```python
from build123d import *

# Parameters (mm, degrees)
F0_W        = 7.62
F0_H        = 17.78
F1_DEPTH    = 12.7
F2_SIZE     = 2.54
F3_R        = 61.3177298103
F4_R        = 76.3155057079
F5_R        = 114.0325409017
F6_T1_DEPTH = 12.7


# Not quite as in the source:
# - a fillet or chamfer that OpenCascade refuses, or shapes differently, is made with other operations: its cross-section is extruded or revolved along the edge and cut away or added


with BuildPart() as f1:
    # F0 (on Front) → F1 (new body)
    with BuildSketch(Plane.XZ):
        with BuildLine():
            Line((-43.3897525072, 184.0122990829), (-43.3897525072, 154.9135648233))
            Line((-43.3897525072, 154.9135648233), (-12.6282460988, 154.9135648233))
            Line((-12.6282460988, 154.9135648233), (-12.6282460988, 184.0122990829))
            Line((-12.6282460988, 184.0122990829), (-23.4354074901, 184.0122990829))
            Line((-23.4354074901, 184.0122990829), (-23.4354074901, 173.8522990829))
            ThreePointArc((-23.4354074901, 173.8522990829), (-24.1793562659, 172.0562478587), (-25.9754074901, 171.3122990829))
            Line((-25.9754074901, 171.3122990829), (-29.7854074901, 171.3122990829))
            ThreePointArc((-29.7854074901, 171.3122990829), (-31.5814587143, 172.0562478587), (-32.3254074901, 173.8522990829))
            Line((-32.3254074901, 173.8522990829), (-32.3254074901, 184.0122990829))
            Line((-32.3254074901, 184.0122990829), (-43.3897525072, 184.0122990829))
        make_face()
        Polygon((-43.3897525072, 154.9135648233), (9.0125808752, 35.5335648233), (34.6665808752, 35.5335648233), (34.6665808752, 53.3135648233), (-12.6282460988, 154.9135648233), align=None)
        with Locations((16.9659831101, 53.1658351564)):
            Rectangle(F0_W, F0_H, mode=Mode.SUBTRACT)
        Polygon((34.6665808752, 35.5335648233), (9.0125808752, 35.5335648233), (9.0125808752, -35.5335648233), (17.9025808752, -35.5335648233), (17.9025808752, 15.2664351767), (25.7765808752, 15.2664351767), (25.7765808752, -35.5335648233), (34.6665808752, -35.5335648233), align=None)
    extrude(amount=F1_DEPTH)

    # F2
    f2_edges = [f1.edges().sort_by_distance(p)[0] for p in [
        (-32.325407, -6.35, 184.012299),
        (-23.435407, -6.35, 184.012299),
        (-12.628246, -6.35, 184.012299),
        (-43.389753, -6.35, 184.012299),
        (17.902581, -6.35, -35.533565),
        (25.776581, -6.35, -35.533565),
        (34.666581, -6.35, -35.533565),
        (9.012581, -6.35, -35.533565),
    ]]
    chamfer(f2_edges, length=F2_SIZE)

    # F3
    f3_edges = [f1.edges().sort_by_distance(p)[0] for p in [
        (34.666581, -6.35, 53.313565),
    ]]
    fillet(f3_edges, radius=F3_R)

    # F4
    f4_edges = [f1.edges().sort_by_distance(p)[0] for p in [
        (-12.628246, -6.35, 154.913565),
    ]]
    fillet(f4_edges, radius=F4_R)

    # F5
    f5_edges = [f1.edges().sort_by_distance(p)[0] for p in [
        (-43.389753, -6.35, 154.913565),
    ]]
    fillet(f5_edges, radius=F5_R)

    # F6: fillet of radius 446.1798259809 on 1 edges, made by hand

    # F6_s2 → F6_t1 (join)
    with BuildSketch(Plane.XZ):
        with BuildLine():
            ThreePointArc((-27.8005344067, 119.3990994032), (-2.6481597508, 44.8323374579), (9.0125808752, -32.9935648233))
            Line((9.0125808752, -32.9935648233), (9.0125808752, 35.5335648233))
            Line((9.0125808752, 35.5335648233), (-27.8005344067, 119.3990994032))
        make_face()
    extrude(amount=F6_T1_DEPTH)


solid = f1.part
```
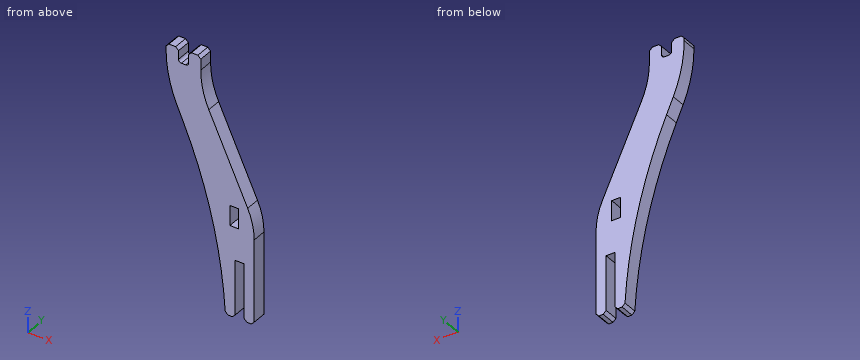
The listing builds one solid part. Answer for the finished solid, in the listing's coordinates (mm). Coordinates: 2 decimals unless noted, no trailing zeros. Loops run counter-clockwise (first coordinate to the right, second up) from the corner with the lowest first, then second, coordinate; pieces in that order, holes last. Notation, with made-up numbers: (89.5, 32) - (96.5, 32) arc R33 cw to (96.5, 68) - close; hole circle Ø6 at (57, -20.75). An arc over 180 degrees is marked (long way). Write item = value, one per line.
1) Section C-C (z = 47) is taken. Determine the outline of the cut face in (x, y).
Responses:
outline = (-3.18, -12.7) - (13.16, -12.7) - (13.16, 0) - (-3.18, 0) - close; (20.78, -12.7) - (34.24, -12.7) - (34.24, 0) - (20.78, 0) - close
2) Each of these flat-tipped pins is pushed along its axis until it touches: P1, Ø4, axis at x = 18.5, y = -6.5, coming from the +Z side; P2, Ø6.5, axis at y = -6, z = 55, coming from the +X side; P3, Ø4, axis at y = -9, z = 51, coming from the -X side. Where does it stop, or does it pass through?
Responses:
P1 = 92.34
P2 = 33.48
P3 = -4.7
3) Section A-A (z = -2.5) is taken. Determine the outline of the cut face in (x, y).
Responses:
outline = (6.11, -12.7) - (17.9, -12.7) - (17.9, 0) - (6.11, 0) - close; (25.78, -12.7) - (34.67, -12.7) - (34.67, 0) - (25.78, 0) - close
4) Find the intervals of material crossed by line 1 along X through (y, z) = (-8, 4); line 2 along X through (y, z) = (-9, 33); line 3 along X through (y, z) = (-8.5, 13) (3 decimals), in increasing order.
Responses:
line_1 = 5.22 to 17.9, 25.78 to 34.67
line_2 = 0.04 to 34.67
line_3 = 3.825 to 17.903, 25.777 to 34.667
5) Section D-D (x = -19) is taken. Determine the outline of the cut face in (y, z), plus the area to 3 significant figures.
Responses:
outline = (-12.7, 97.84) - (0, 97.84) - (0, 184.01) - (-12.7, 184.01) - close
area = 1,090 mm^2
